The listing builds one solid part. Answer for the finished solid, in the listing's coordinates (mm). Face numbers are marked on the shaded views. Give positions to 0.01 mm unless a question says otherwise; leave off trailing zeros. Loops run counter-clockwise (first coordinate to the right, second up) from the corner with the lowest first, then second, coordinate; pieces in that order, holes last.
Item 1: Section D-D, the plane x = -35 is taken. Give the vertices of the cut face in (y, z).
Item 2: This flat-tipped pin is pushed along its axis until it touches: pin 1 Ø5 at (x, z) = (13, 9.5) entering from +Y. Where does it stop, or does it pass through?
Item 3: Section A-A, the plane x = -50 is taken. Give the vertices of the cut face in (y, z).
Item 4: Section B-B, the plane z = 9.25 is taken. Give the number of separate pieces and of enclosed holes in the cut face, and give its area (3 significant figures).
Item 5: The mould has two halves that part along Z. Classify the marked faces 1, 2 and 3: pulls with the +Z half, pulls with the -Z half, needs draft (parallel to the pull), parting line crosses it, or undercut.
Item 6: Section C-C, the plane x = 52 is taken. Give the vertices of the cut face in (y, z), and give its area (3 significant figures).
Item 7: Consider line 1 along Y through (x, z) = (52, 4.5); line 2 along X through (y, z) = (-34, 8.25); line 3 along Y through (x, z) = (-50, 3). Determine where each line is inside the solid, lowest interval first.
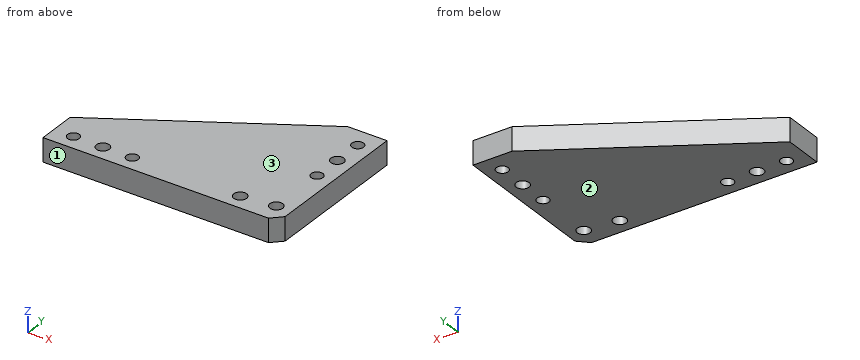
from build123d import *

# Parameters (mm, degrees)
SKETCH_1_W         = 120
SKETCH_1_H         = 80
EXTRUDE_1_DEPTH    = 12
CHAMFER_1_SIZE     = 100
CHAMFER_1_SIZE2    = 60
CHAMFER_2_SIZE     = 5
MM_1_D             = 6
HOLE_WIZARD_M6_1_D = 6.6


with BuildPart() as part:
    # 草图1 → 凸台-拉伸1 (new body)
    with BuildSketch(Plane.XY):
        Rectangle(SKETCH_1_W, SKETCH_1_H)
    extrude(amount=EXTRUDE_1_DEPTH)

    # 倒角1
    chamfer_1_edges = [part.edges().sort_by_distance(p)[0] for p in [
        (-60, 40, 6),
    ]]
    chamfer_1_side = [part.faces().sort_by_distance(p)[0] for p in [
        (0, 40, 6),
    ]]
    chamfer(chamfer_1_edges, length=CHAMFER_1_SIZE, length2=CHAMFER_1_SIZE2, reference=chamfer_1_side[0])

    # 倒角2
    chamfer_2_edges = [part.edges().sort_by_distance(p)[0] for p in [
        (60, -40, 6),
    ]]
    chamfer(chamfer_2_edges, length=CHAMFER_2_SIZE)

    # 大小mm 暗销孔1 (through all)
    with Locations(Plane(origin=(0, 0, 0), x_dir=(-1, 0, 0), z_dir=(0, 0, -1))):
        with Locations((50, -32), (20, -32), (-52, 30), (-52, 0)):
            Hole(MM_1_D / 2)

    # M6 间隙孔1 (through all)
    with Locations(Plane(origin=(0, 0, 0), x_dir=(-1, 0, 0), z_dir=(0, 0, -1))):
        with Locations((-52, 15), (-52, -30), (-35, -32), (35, -32)):
            Hole(HOLE_WIZARD_M6_1_D / 2)


solid = part.part
Worked answers:
1. outline: (-40, 0) - (-35.3, 0) - (-35.3, 12) - (-40, 12) - close; (-28.7, 0) - (-5, 0) - (-5, 12) - (-28.7, 12) - close
2. pin 1: stops at y = 25.3
3. outline: (-40, 0) - (-35, 0) - (-35, 12) - (-40, 12) - close; (-29, 0) - (-14, 0) - (-14, 12) - (-29, 12) - close
4. separate pieces: 1
4. enclosed holes: 8
4. area: 6,340 mm2
5. face 1: needs draft
5. face 2: pulls with the -Z half
5. face 3: pulls with the +Z half
6. outline: (-40, 0) - (-33.3, 0) - (-33.3, 12) - (-40, 12) - close; (-26.7, 0) - (-3, 0) - (-3, 12) - (-26.7, 12) - close; (3, 0) - (11.7, 0) - (11.7, 12) - (3, 12) - close; (18.3, 0) - (27, 0) - (27, 12) - (18.3, 12) - close; (33, 0) - (40, 0) - (40, 12) - (33, 12) - close
6. area: 658 mm2
7. line 1: y = -40 to -33.3, -26.7 to -3, 3 to 11.7, 18.3 to 27, 33 to 40
7. line 2: x = -60 to -52.24, -47.76 to -37.62, -32.38 to -22.24, -17.76 to 32.38, 37.62 to 60
7. line 3: y = -40 to -35, -29 to -14
